```python
from build123d import *


with BuildPart() as part:
    # Croquis1 → Revolución1 (revolve)
    with BuildSketch(Plane.XY, mode=Mode.PRIVATE) as revoluci_n1_sk:
        with BuildLine():
            Line((49.909918854, 0), (55.409918854, 0))
            Line((55.409918854, 0), (55.409918854, 3))
            Line((55.409918854, 3), (51.759057178, 3))
            ThreePointArc((51.759057178, 3), (50.414552694, 3.51935565), (49.76832421, 4.807692308))
            ThreePointArc((49.76832421, 4.807692308), (33.612612102, 37.016108759), (0, 50))
            Line((0, 50), (0, 47))
            ThreePointArc((0, 47), (32.221576622, 34.21651648), (46.915323723, 2.82))
            ThreePointArc((46.915323723, 2.82), (47.853222474, 0.815967033), (49.909918854, 0))
        make_face()
    revolve(revoluci_n1_sk.sketch.rotate(Axis((0, 0, 0), (0, 1, 0)), 90), axis=Axis((0, 0, 0), (0, 1, 0)))


solid = part.part
```
CAD build for the part. Positions are in the model's coordinates, mm. Give positions to 0.01 mm unless a question says otherwise; leave off trailing zeros. Order: outer loops, then holes, each group sorted by start corner. A loop starts at its lowest first (then second) coordinate and runs counter-clockwise, first axis right, second up.
(1) Mould opens along Z. For faces 1 (the flat face through (-8, 0, -50)), 2 (the cylindrical face through (21.222, 1.521, -51.185)) say: released by +Z, released by -Z, zero draft, split by the parting line, or undercut.
(2) Saw through at C-C, the plane y = 11. Give the cut face in (x, z) (3 decimals).
(3) Flat gauge pins, fed straight in: pin 1 (12 mm diameter, centred on y = 15.5, z = 9, fed in from -X); pin 2 (10 mm diameter, centred on x = -5, z = -20, fed in from +Y); pin 3 (5 mm diameter, centred on y = 19, z = 21.5, fed in from -X). Where does each tip first touch, or does it go through?
(4) Drill centre lines: L1, parallel to X at y = 29, z = -5; L2, parallel to X at y = 27, z = -10; L3, parallel to Z at x = -28, y = 12. Where is each one in solid material? Low to high.
Results found:
1. face 1: zero draft
1. face 2: split by the parting line
2. outline: circle Ø97.55 at (0, 0); hole circle Ø91.389 at (0, 0)
3. pin 1: stops at x = -48.56
3. pin 2: stops at y = 47.5
3. pin 3: stops at x = -42.59
4. L1: x = -40.42 to -36.65, 36.65 to 40.42
4. L2: x = -40.88 to -37.15, 37.15 to 40.88
4. L3: z = -39.65 to -35.79, 35.79 to 39.65
